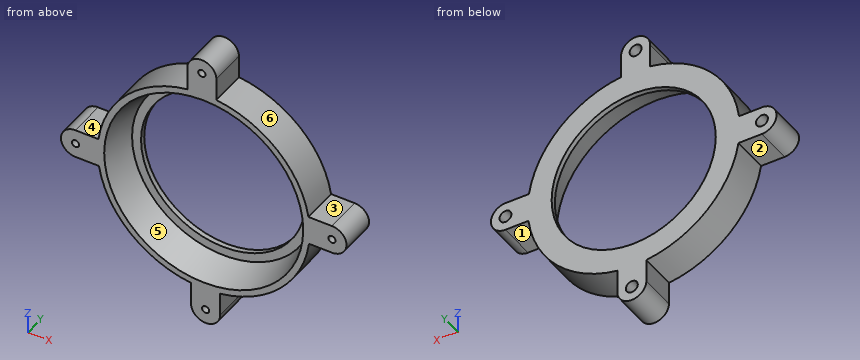
```python
from build123d import *

# Parameters (mm, degrees)
SKETCH1_R           = 62
SKETCH1_R_2         = 58.2
BOSS_EXTRUDE1_DEPTH = 18.4
BOSS_EXTRUDE1_DRAFT = -15
SKETCH2_R           = 82
SKETCH2_R_2         = 62
CUT_EXTRUDE1_DEPTH  = 97.425519359
SKETCH3_R           = 62
SKETCH3_R_2         = 48
BOSS_EXTRUDE2_DEPTH = 3
SKETCH4_R           = 2.125
BOSS_EXTRUDE3_DEPTH = 21.4
CIRPATTERN1_COUNT   = 4
SKETCH5_R           = 3.5
CUT_EXTRUDE2_DEPTH  = 9.4


with BuildPart() as part:
    # Sketch1 → Boss-Extrude1 (with draft: the straight prism first)
    with BuildSketch(Plane(origin=(0, 0, 0), x_dir=(1, 0, 0), z_dir=(0, 1, 0))):
        Circle(SKETCH1_R)
        Circle(SKETCH1_R_2, mode=Mode.SUBTRACT)
    extrude(amount=BOSS_EXTRUDE1_DEPTH)
    # Boss-Extrude1: the draft: its side faces are tilted about the plane it starts from
    boss_extrude1_sides = [part.faces().sort_by_distance(p)[0] for p in [
        (-62, 9.2, 0),
        (-58.2, 9.2, 0),
    ]]
    draft(boss_extrude1_sides, Plane(origin=(0, 0, 0), x_dir=(1, 0, 0), z_dir=(0, 1, 0)), BOSS_EXTRUDE1_DRAFT)

    # Sketch2 → Cut-Extrude1 (cut, through all)
    with BuildSketch(Plane.XZ):
        Circle(SKETCH2_R)
        with Locations(Location((0, 0, 0), (0, 0, 270))):
            Circle(SKETCH2_R_2, mode=Mode.SUBTRACT)
    extrude(amount=-CUT_EXTRUDE1_DEPTH, mode=Mode.SUBTRACT)

    # Sketch3 → Boss-Extrude2 (add)
    with BuildSketch(Plane(origin=(0, 18.4, 0), x_dir=(1, 0, 0), z_dir=(0, 1, 0))):
        with Locations(Location((0, 0, 0), (0, 0, 90))):
            Circle(SKETCH3_R)
        with Locations(Location((0, 0, 0), (0, 0, 270))):
            Circle(SKETCH3_R_2, mode=Mode.SUBTRACT)
    extrude(amount=BOSS_EXTRUDE2_DEPTH)

    # Sketch4 → Boss-Extrude3 (add)
    with BuildSketch(Plane(origin=(0, 21.4, 0), x_dir=(1, 0, 0), z_dir=(0, 1, 0))):
        with BuildLine():
            Line((-75, 9.610336935), (-58.480915803, 9.610336935))
            Line((-58.480915803, 9.610336935), (-58.480915803, -7.389663065))
            Line((-58.480915803, -7.389663065), (-75, -7.389663065))
            ThreePointArc((-75, -7.389663065), (-83.5, 1.110336935), (-75, 9.610336935))
        make_face()
        with Locations(Location((-75, 1.110336935, 0), (0, 0, 270))):
            Circle(SKETCH4_R, mode=Mode.SUBTRACT)
    boss_extrude3 = extrude(amount=-BOSS_EXTRUDE3_DEPTH)

    # CirPattern1: Boss-Extrude3 ×4 about axis
    cirpattern1_axis = Axis((0, 0, 0), (0, 1, 0))
    for i in range(1, CIRPATTERN1_COUNT):
        add(boss_extrude3.rotate(cirpattern1_axis, i * 360 / CIRPATTERN1_COUNT))

    # Sketch5 → Cut-Extrude2 (cut)
    with BuildSketch(Plane(origin=(0, 21.4, 0), x_dir=(1, 0, 0), z_dir=(0, 1, 0))):
        with Locations(Location((-75, 1.110336935, 0), (0, 0, 270))):
            Circle(SKETCH5_R)
        with Locations(Location((1.110336935, 75, 0), (0, 0, 270))):
            Circle(SKETCH5_R)
        with Locations(Location((75, -1.110336935, 0), (0, 0, 270))):
            Circle(SKETCH5_R)
        with Locations(Location((-1.110336935, -75, 0), (0, 0, 270))):
            Circle(SKETCH5_R)
    extrude(amount=-CUT_EXTRUDE2_DEPTH, mode=Mode.SUBTRACT)


solid = part.part
```
Verification items for the finished model (mm, model axes). Face numbers are marked on the shaded views. A direction names the side the tool comes from. Round coordinates to 2 decimals unless told otherwise and drop trailing zeros. Write each loop counter-clockwise with the first axis right and the second up, starting at its lowest first coordinate (ties: lowest second). Pieces come first, ordered by that corner, then holes.
1. Section check A-A on y = 6.25. Enter the section's corners in (x, z) (3 decimals), plus the area to 3 significant figures.
2. Section check B-B on z = 66.5. Enter the section's corners in (x, y), plus the area to 3 significant figures.
3. Scan lines: L1, parallel to X at y = 16.5, z = 75; L2, parallel to X at y = 3.5, z = 2.5; L3, parallel to Z at x = 75, y = 6.25. Record each from-to range of solid material in increasing order.
4. Draft check along X on the marked faces 4, 5 and 6. Enter one of: +X half, -X half, draft (parallel to the pull), parting line (faces both ways), or undercut.
5. Access from +Z, -Z, +X, -X, +Y, -Y to the whole of each face (thin tool, end or side, straight path). Record for the marked faces 1, 2 and 3.
6. Gauge pin test, flat ends, axial feed: P1, Ø4, axis at y = 15, z = -71, coming from the +X side; P2, Ø7, axis at x = 70.5, y = 15, coming from the +Z side; P3, Ø1, axis at x = -11, y = 6.5, coming from the -Z side; P4, Ø2.5, axis at x = 75, z = 1.11, coming from the -Y side. Record the tip position at first contact, or that the pin passes through.
Answer:
1. outline: (-75, -9.61) - (-61.251, -9.61) arc R62 ccw to (-7.39, -61.558) - (-7.39, -75) arc R8.5 ccw to (9.61, -75) - (9.61, -61.251) arc R62 ccw to (61.558, -7.39) - (75, -7.39) arc R8.5 ccw to (75, 9.61) - (61.251, 9.61) arc R62 ccw to (7.39, 61.558) - (7.39, 75) arc R8.5 ccw to (-9.61, 75) - (-9.61, 61.251) arc R62 ccw to (-61.558, 7.39) - (-75, 7.39) arc R8.5 ccw to start; hole circle Ø4.25 at (-75, -1.11); hole circle Ø113.051 at (0, 0); hole circle Ø4.25 at (-1.11, 75); hole circle Ø4.25 at (1.11, -75); hole circle Ø4.25 at (75, 1.11)
1. area: 3,330 mm2
2. outline: (-9.61, 0) - (7.39, 0) - (7.39, 21.4) - (-9.61, 21.4) - close
2. area: 364 mm2
3. L1: x = -9.61 to -4.61, 2.39 to 7.39
3. L2: x = -82.7 to -57.21, 57.21 to 73.39, 76.61 to 83.39
3. L3: z = -7.39 to -1.01, 3.24 to 9.61
4. face 4: draft
4. face 5: undercut
4. face 6: +X half
5. face 1: -Z, +X, +Y, -Y
5. face 2: -Z, -X, +Y, -Y
5. face 3: +Z, +X, +Y, -Y
6. P1: stops at x = 9.61
6. P2: stops at z = 9.61
6. P3: stops at z = -61.1
6. P4: passes through
